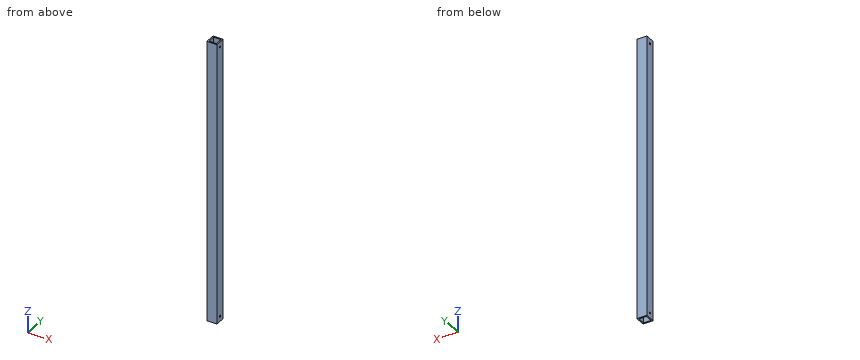
Autodesk Inventor part; units mm, degrees
ref_plane "YZ Plane" through (0, 0, 0) normal (1, 0, 0) x (0, 1, 0)
ref_plane "XZ Plane" through (0, 0, 0) normal (0, 1, 0) x (-1, 0, 0)
ref_plane "XY Plane" through (0, 0, 0) normal (0, 0, 1) x (1, 0, 0)
sketch "Sketch1" plane through (0, 0, 0) normal (0, 0, 1) x (1, 0, 0)
  line L0 (0, 0) -> (25.4, 0)
  line L1 (25.4, 0) -> (25.4, 25.4)
  line L2 (25.4, 25.4) -> (0, 25.4)
  line L3 (0, 25.4) -> (0, 0)
  line L4 (3.175, 22.225) -> (22.225, 22.225)
  line L5 (22.225, 22.225) -> (22.225, 3.175)
  line L6 (22.225, 3.175) -> (3.175, 3.175)
  line L7 (3.175, 3.175) -> (3.175, 22.225)
  dimension "d0" = 25.4
  dimension "d1" = 25.4
  dimension "d2" = 3.175
extrude "Extrusion1" add sketch "Sketch1" along normal blind 711.2
sketch "Sketch2" plane through (25.4, 0, 0) normal (1, 0, 0) x (0, 0, -1)
  line L0 (0, 3.175) -> (0, 22.225) construction
  line L1 (0, 12.7) -> (-12.7, 12.7) construction
  line L2 (-711.2, 22.225) -> (-711.2, 3.175) construction
  line L3 (-711.2, 12.7) -> (-698.5, 12.7) construction
  circle A0 centre (-698.5, 12.7) radius 2.5797
  circle A1 centre (-12.7, 12.7) radius 2.5797
  point P0 (0, 0)
  dimension "d5" = 12.7
  dimension "d6" = 12.7
  dimension "d7" = 5.1594
extrude "Extrusion2" cut sketch "Sketch2" against normal blind 25.4
properties part number "1x1 28 in"
Part model, mm, in its own coordinate system. Coordinates: 2 decimals unless noted, no trailing zeros. Order: outer loops, then holes, each group sorted by start corner. A loop starts at its lowest first (then second) coordinate and runs counter-clockwise, first axis right, second up. Notation, with made-up numbers: M -39.75,89 L 7.25,89 A19 ccw 7.25,101 Z; hole C -31,-6.5 d1. An arc over 180 degrees is marked long. Use a Markdown table: item, result.
(1) Cut at B-B on z = 403.5. Write the cut outline in (x, y) (3 decimals).
A:
| item | result |
|---|---|
| outline | M 0,0 L 25.4,0 L 25.4,25.4 L 0,25.4 Z; hole M 3.175,3.175 L 22.225,3.175 L 22.225,22.225 L 3.175,22.225 Z |
(2) Probe L1, parallel to X at y = 4.5, z = 487 (3 decimals); L2, parallel to Y at x = 1.6, z = 698.5. List the from-to ranges inside material, lowest first.
A:
| item | result |
|---|---|
| L1 | x = 0 to 3.175, 22.225 to 25.4 |
| L2 | y = 0 to 10.12, 15.28 to 25.4 |
(3) Cut at A-A on x = 10.5. Write the cut outline in (y, z) (3 decimals), then the cut area to 3 significant figures.
A:
| item | result |
|---|---|
| outline | M 0,0 L 3.175,0 L 3.175,711.2 L 0,711.2 Z; M 22.225,0 L 25.4,0 L 25.4,711.2 L 22.225,711.2 Z |
| area | 4,520 mm^2 |
